Geometry: final body of the model. Coordinates: model frame, mm. Face numbers are marked on the shaded views. A direction names the side the tool comes from. Round coordinates to 2 decimals unless told otherwise and drop trailing zeros. Write each loop counter-clockwise with the first axis right and the second up, starting at its lowest first coordinate (ties: lowest second). Pieces come first, ordered by that corner, then holes. Notation, with made-up numbers: (-28.75, 79.25) - (1.25, 79.25) arc R28 cw to (1.25, 113.25) - close; hole circle Ø9 at (-36, 14). An arc over 180 degrees is marked (long way). Write each question's results on one line, items separated by ' | '.
from build123d import *

# Parameters (mm, degrees)
F0_W     = 57.15
F0_H     = 50.8
F1_DEPTH = 6.35
F2_W     = 6.35
F2_H     = 50.8
F3_DEPTH = 203.2
F4_R     = 12.7
F5_DEPTH = 6.35
F7_R     = 6.35
F8_DEPTH = 101.6


with BuildPart() as f1:
    # F0 (on Top) → F1 (new body)
    with BuildSketch(Plane.XY):
        with Locations((-28.575, 0)):
            Rectangle(F0_W, F0_H)
    extrude(amount=F1_DEPTH)

    # F2 (on face) → F3 (join)
    with BuildSketch(Plane.XY.offset(6.35)):
        with Locations((-53.975, 0)):
            Rectangle(F2_W, F2_H)
    extrude(amount=F3_DEPTH)

    # F4 (on face) → F5 (cut, through all)
    with BuildSketch(Plane(origin=(-57.15, 0, 0), x_dir=(0, -1, 0), z_dir=(-1, 0, 0))):
        with Locations((0, 107.95)):
            Circle(F4_R)
    extrude(amount=-F5_DEPTH, mode=Mode.SUBTRACT)

    # F6: F1 across plane


with BuildPart() as f1_1:
    add(f1.part)
    add(f1.part.mirror(Plane.YZ))

    # F7 (on face) → F8 (join, through all)
    with BuildSketch(Plane.YZ.offset(-50.8)):
        with Locations((0, 196.85)):
            Circle(F7_R)
    extrude(amount=F8_DEPTH)


solid = f1_1.part
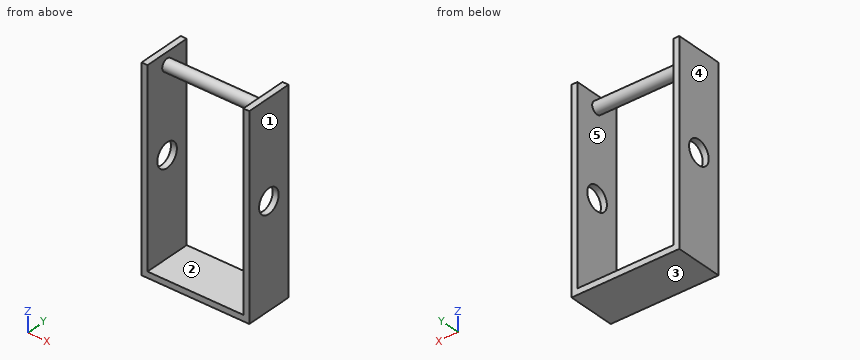
Q1. Mould query, pull axis Z, two halves, no side actions, for the marked faces 3, 4 and 5. Classes: pulls with the +Z half, pulls with the -Z half, needs draft (parallel to the pull), parting line crosses it, or undercut.
Answer block:
face 3: pulls with the -Z half | face 4: needs draft | face 5: undercut
Q2. Section query A-A, the plane z = 37. Return loops of the section in (x, y).
Answer block:
outline: (-57.15, -25.4) - (-50.8, -25.4) - (-50.8, 25.4) - (-57.15, 25.4) - close; (50.8, -25.4) - (57.15, -25.4) - (57.15, 25.4) - (50.8, 25.4) - close
Q3. Section query C-C, the plane y = 0. Return loops of the section in (x, z).
Answer block:
outline: (-57.15, 0) - (57.15, 0) - (57.15, 95.25) - (50.8, 95.25) - (50.8, 6.35) - (-50.8, 6.35) - (-50.8, 95.25) - (-57.15, 95.25) - close; (-57.15, 120.65) - (-50.8, 120.65) - (-50.8, 190.5) - (50.8, 190.5) - (50.8, 120.65) - (57.15, 120.65) - (57.15, 209.55) - (50.8, 209.55) - (50.8, 203.2) - (-50.8, 203.2) - (-50.8, 209.55) - (-57.15, 209.55) - close
Q4. Access query for the marked faces 1 and 2. Directions: +Z, -Z, +X, -X, +Y, -Y. A direction counts if a zero-diameter tool reaches every point of the face in a straight line with its end or side. Return the directions, or none.
Answer block:
face 1: +Z, -Z, +X, +Y, -Y | face 2: +Y, -Y
Q5. Section query B-B, the plane z = 107.95. Return loops of the section in (x, y).
Answer block:
outline: (-57.15, -25.4) - (-50.8, -25.4) - (-50.8, -12.7) - (-57.15, -12.7) - close; (-57.15, 12.7) - (-50.8, 12.7) - (-50.8, 25.4) - (-57.15, 25.4) - close; (50.8, -25.4) - (57.15, -25.4) - (57.15, -12.7) - (50.8, -12.7) - close; (50.8, 12.7) - (57.15, 12.7) - (57.15, 25.4) - (50.8, 25.4) - close
Q6. Section query D-D, the plane x = -35.5. Return loops of the section in (y, z).
Answer block:
outline: (-25.4, 0) - (25.4, 0) - (25.4, 6.35) - (-25.4, 6.35) - close; circle Ø12.7 at (0, 196.85)
Q7. Ray query, line 1 along X through (y, z) = (-16, 119.5); line 2 along Z through (x, y) = (-54, 0); line 3 along Y through (x, z) = (-54, 107). Return the intervals inside material, ascending.
Answer block:
line 1: -57.15 to -50.8, 50.8 to 57.15 | line 2: 0 to 95.25, 120.65 to 209.55 | line 3: -25.4 to -12.66, 12.66 to 25.4
